Design review of the part built by this model. Coordinates are the model's own, in mm. Round coordinates to 2 decimals unless told otherwise and drop trailing zeros. Order: outer loops, then holes, each group sorted by start corner. A loop starts at its lowest first (then second) coordinate and runs counter-clockwise, first axis right, second up. Notation, with made-up numbers: (35, -15) - (83, -15) arc R10 cw to (83, -7) - close; hole circle Ø7 at (20.5, 11). An arc over 180 degrees is marked (long way). Write item = value, one per line.
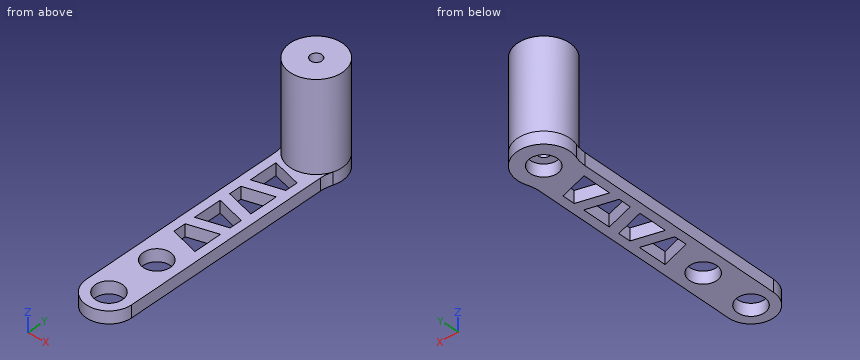
from build123d import *

# Parameters (mm, degrees)
SKETCH1_R           = 7.75
BOSS_EXTRUDE1_DEPTH = 7
SKETCH2_R           = 15
SKETCH2_R_2         = 3.25
BOSS_EXTRUDE2_DEPTH = 51


with BuildPart() as part:
    # Sketch1 → Boss-Extrude1 (new body)
    with BuildSketch(Plane.XY):
        with BuildLine():
            Line((-14.121781939, 65.817369233), (-14.121781939, -52.520726978))
            ThreePointArc((-14.121781939, -52.520726978), (-1.121781939, -65.520726978), (11.878218061, -52.520726978))
            Line((11.878218061, -52.520726978), (11.878218061, 65.817369233))
            ThreePointArc((11.878218061, 65.817369233), (12.166002849, 69.197986251), (13.021075204, 72.481314255))
            ThreePointArc((13.021075204, 72.481314255), (-1.121781939, 92.479273022), (-15.264639082, 72.481314255))
            ThreePointArc((-15.264639082, 72.481314255), (-14.409566727, 69.197986251), (-14.121781939, 65.817369233))
        make_face()
        with Locations((-1.121781939, -52.520726978)):
            Circle(SKETCH1_R, mode=Mode.SUBTRACT)
        with Locations((-1.121781939, -22.520726978)):
            Circle(SKETCH1_R, mode=Mode.SUBTRACT)
        with Locations((-1.121781939, 77.479273022)):
            Circle(SKETCH1_R, mode=Mode.SUBTRACT)
        Polygon((-9.121781939, 3.957653989), (-9.121781939, -3.042346011), (6.878218061, -7.32953309), (6.878218061, 8.67046691), align=None, mode=Mode.SUBTRACT)
        Polygon((-9.121781939, 31.957653989), (6.878218061, 27.67046691), (6.878218061, 43.67046691), (-9.121781939, 38.957653989), align=None, mode=Mode.SUBTRACT)
        Polygon((6.878218061, 56.67046691), (-9.121781939, 60.957653989), (-9.121781939, 44.957653989), (6.878218061, 49.67046691), align=None, mode=Mode.SUBTRACT)
        Polygon((-9.121781939, 9.957653989), (6.878218061, 14.67046691), (6.878218061, 21.67046691), (-9.121781939, 25.957653989), align=None, mode=Mode.SUBTRACT)
    extrude(amount=BOSS_EXTRUDE1_DEPTH)

    # Sketch2 → Boss-Extrude2 (add)
    with BuildSketch(Plane.XY.offset(7)):
        with Locations(Location((-1.121781939, 77.479273022, 0), (0, 0, 199.462950946))):
            Circle(SKETCH2_R)
        with Locations((-1.121781939, 77.479273022)):
            Circle(SKETCH2_R_2, mode=Mode.SUBTRACT)
    extrude(amount=BOSS_EXTRUDE2_DEPTH)


solid = part.part
Item 1: Take a section at C-C, the plane z = 27.5. State the section outline as (x, y) points.
Data:
outline = circle Ø30 at (-1.12, 77.48); hole circle Ø6.5 at (-1.12, 77.48)
Item 2: For line 1 along Z through (x, y) = (8.5, -43); line 2 along Y through (x, z) = (0, 38.5); line 3 along X through (y, z) = (73.5, 31), list the stretches that pass through material, from the lowest coordinate up. Write a range as [from, to].
Data:
line_1 = [0, 7]
line_2 = [62.52, 74.43], [80.53, 92.44]
line_3 = [-15.58, 13.34]
Item 3: Take a section at B-B, the plane y = -48. State the section outline as (x, z) points.
Data:
outline = (-14.12, 0) - (-7.42, 0) - (-7.42, 7) - (-14.12, 7) - close; (5.17, 0) - (11.88, 0) - (11.88, 7) - (5.17, 7) - close
Item 4: Take a section at A-A, the plane x = -7.5. Count the separate pieces of the cut face and the enclosed holes in it, and give its area (3 significant figures).
Data:
separate_pieces = 7
enclosed_holes = 0
area = 1,960 mm2
Item 5: Insertion check: P1, Ø2, axis at y = 34, z = 4, coming from the -X side; P2, Ø2, axis at y = 34, z = 2, coming from the +X side; P3, Ø5, axis at x = 8.5, z = 40, coming from the +Y side; P4, Ø2, axis at x = -8, y = 48, coming from the -Z side. Each pin has a flat end and moves straight along its axis. Give the tip position at first contact, or say it passes through.
Data:
P1 = -14.12
P2 = 11.88
P3 = 90.68
P4 = through
